Job drawing, mm, ordinate dimensions from the low corner. One solid piece. A direction names the side the tool comes from. Coordinates: 2 decimals unless noted, no trailing zeros. Order: outer loops, then holes, each group sorted by start corner. A loop starts at its lowest first (then second) coordinate and runs counter-clockwise, first axis right, second up. Notation, with made-up numbers: (-31.75, 82) - (23.25, 82) arc R31 ccw to (23.25, 120) - close; hole circle Ø5 at (-34, -26.5). An arc over 180 degrees is marked (long way). Write each question's results on one line, items separated by ' | '. Start each with the question number.
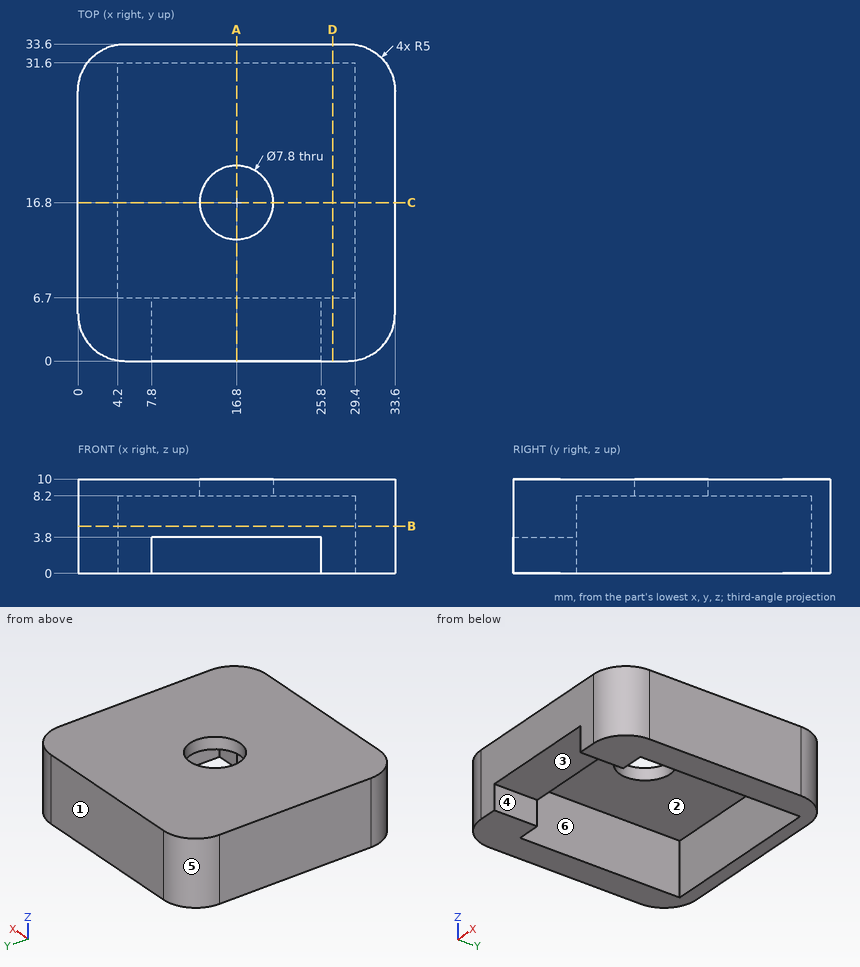
Item 1: Slice it at D-D (x = 27). Write the cut outline in (y, z), then the cut area to 3 significant figures.
Item 2: Which spindle directions (+Z, -Z, +X, -X, +Y, -Y) get a long thin tool onto all of the face, cutting with end or side? Do the marked faces 1, 2 and 3. Say none if no direction does.
Item 3: Slice it at B-B (z = 5). Write the cut outline in (x, y), then the cut area to 3 significant figures.
Item 4: Probe probe 1 along Y at (x, z) = (16.8, 8.6); probe 2 along X at (y, z) = (19.5, 4.5); probe 3 along Y at (x, z) = (8, 4.5). List the from-to ranges inside material, lowest first.
Item 5: Pull direction Y, two halves, no side cores. Call the marked faces 4, 5 and 6: released by +Y, released by -Y, zero draft, split by the parting line, or undercut.
Item 6: Slice it at C-C (y = 16.8). Write the cut outline in (x, z), then the cut area to 3 significant figures.
Item 7: Flat gauge pins, fed straight in: P1, Ø7.5, axis at x = 15.5, y = 24, coming from the -Z side; P2, Ø7.5, axis at x = 19.5, y = 4, coming from the -Z side; P3, Ø4, axis at y = 2, z = 1, coming from the -X side. Where does each tip first touch, or does it go through?
Item 8: Slice it at A-A (x = 16.8). Write the cut outline in (y, z), then the cut area to 3 significant figures.
Resolved:
1) outline: (0, 0) - (6.7, 0) - (6.7, 8.2) - (31.6, 8.2) - (31.6, 0) - (33.6, 0) - (33.6, 10) - (0, 10) - close | area: 132 mm^2
2) face 1: +Z, -Z, +X, -X, +Y | face 2: -Z | face 3: -Z, -Y
3) outline: (0, 5) arc R5 ccw to (5, 0) - (28.6, 0) arc R5 ccw to (33.6, 5) - (33.6, 28.6) arc R5 ccw to (28.6, 33.6) - (5, 33.6) arc R5 ccw to (0, 28.6) - close; hole (4.2, 6.7) - (29.4, 6.7) - (29.4, 31.6) - (4.2, 31.6) - close | area: 480 mm^2
4) probe 1: 0 to 12.9, 20.7 to 33.6 | probe 2: 0 to 4.2, 29.4 to 33.6 | probe 3: 0 to 6.7, 31.6 to 33.6
5) face 4: zero draft | face 5: released by +Y | face 6: undercut
6) outline: (0, 0) - (4.2, 0) - (4.2, 8.2) - (12.9, 8.2) - (12.9, 10) - (0, 10) - close; (20.7, 8.2) - (29.4, 8.2) - (29.4, 0) - (33.6, 0) - (33.6, 10) - (20.7, 10) - close | area: 115 mm^2
7) P1: z = 8.2 | P2: z = 3.8 | P3: x = 0.1
8) outline: (0, 3.8) - (6.7, 3.8) - (6.7, 8.2) - (12.9, 8.2) - (12.9, 10) - (0, 10) - close; (20.7, 8.2) - (31.6, 8.2) - (31.6, 0) - (33.6, 0) - (33.6, 10) - (20.7, 10) - close | area: 92.3 mm^2
